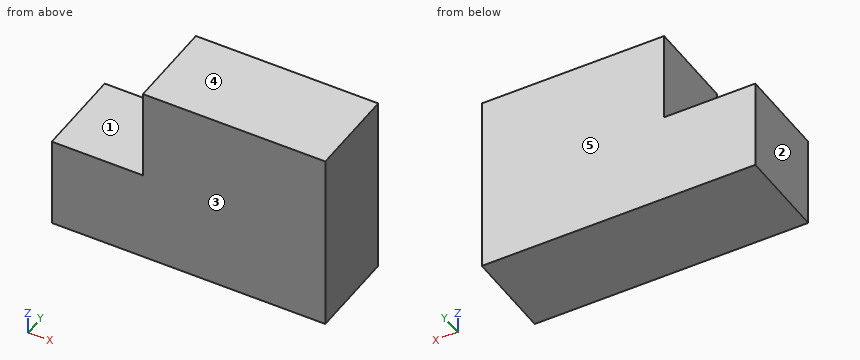
from build123d import *

# Parameters (mm, degrees)
F0_W     = 19.05
F0_H     = 19.05
F1_DEPTH = 19.05


with BuildPart() as f1:
    # F0 (on Front) → F1 (new body)
    with BuildSketch(Plane.XZ):
        Rectangle(F0_W, F0_H)
        with Locations((19.05, 0)):
            Rectangle(F0_W, F0_H)
        with Locations((19.05, 19.05)):
            Rectangle(F0_W, F0_H)
        with Locations((0, 19.05)):
            Rectangle(F0_W, F0_H)
        with Locations((-19.05, 0)):
            Rectangle(F0_W, F0_H)
    extrude(amount=F1_DEPTH)


solid = f1.part
The model under review builds one solid part; all positions refer to its coordinate system, in mm. Face numbers are marked on the shaded views. A direction names the side the tool comes from. Round coordinates to 2 decimals unless told otherwise and drop trailing zeros. Loops run counter-clockwise (first coordinate to the right, second up) from the corner with the lowest first, then second, coordinate; pieces in that order, holes last. Notation, with made-up numbers: (85, 34) -> (136, 34) arc R22 ccw to (136, 63) -> close; hole circle Ø8 at (-24.75, 71). An arc over 180 degrees is marked (long way). Answer as CSV lines item,"result".
1) Add section A-A on y = -7. Write out the cut boundary in (x, z) (3 decimals).
Geometry results:
outline,"(-28.575, -9.525) -> (28.575, -9.525) -> (28.575, 28.575) -> (-9.525, 28.575) -> (-9.525, 9.525) -> (-28.575, 9.525) -> close"
2) Tool access review of the marked faces 1 and 2: name each direction out of +Z, -Z, +X, -X, +Y, -Y from which nothing blocks a thin tool from reaching the whole face with its end or side.
Geometry results:
face 1,"+Z, -X, +Y, -Y"
face 2,"+Z, -Z, -X, +Y, -Y"
3) Draft analysis for pull direction Y (two halves, no side actions). For the marked faces 3, 4 and 5, state which applies: pulls with the +Y half, pulls with the -Y half, needs draft (parallel to the pull), parting line crosses it, or undercut.
Geometry results:
face 3,"pulls with the -Y half"
face 4,"needs draft"
face 5,"pulls with the +Y half"
4) For P1, Ø6, axis at y = -3.5, z = 19, coming from the -X side (3 decimals); P2, Ø8, axis at x = -14.5, y = -8, coming from the +Z side (3 decimals), all flat-tipped, find the tip position at first contact; note any pin that passes through.
Geometry results:
P1,"stops at x = -9.525"
P2,"stops at z = 9.525"
5) To check wall thickness, follow line 1 along X through (y, z) = (-14.5, 17) (3 decimals); line 2 along Z through (x, y) = (-19, -9.5) (3 decimals). State the ranges of each line that lie inside material, in increasing order. Write a range as from..to.
Geometry results:
line 1,"x = -9.525..28.575"
line 2,"z = -9.525..9.525"
6) Add section B-B on x = -13.5. Write out the cut boundary in (y, z) (3 decimals), plus the area to 3 significant figures.
Geometry results:
outline,"(-19.05, -9.525) -> (0, -9.525) -> (0, 9.525) -> (-19.05, 9.525) -> close"
area,"363 mm²"
